```python
from build123d import *

# Parameters (mm, degrees)
ESQUISSE1_W             = 330
ESQUISSE1_H             = 220
BOSS_EXTRU_1_DEPTH      = 6
ESQUISSE3_W             = 20
ESQUISSE3_H             = 6
ESQUISSE3_W_2           = 30
ESQUISSE3_W_3           = 6
ESQUISSE3_H_2           = 10
ENL_V_MAT_EXTRU_2_DEPTH = 6
ESQUISSE4_R             = 1.4
ENL_V_MAT_EXTRU_3_DEPTH = 6


with BuildPart() as part:
    # Esquisse1 → Boss.-Extru.1 (new body)
    with BuildSketch(Plane.XY):
        Rectangle(ESQUISSE1_W, ESQUISSE1_H)
    extrude(amount=BOSS_EXTRU_1_DEPTH)

    # Esquisse3 → Enlèv. mat.-Extru.2 (cut)
    with BuildSketch(Plane.XY.offset(6)):
        with Locations((-125, 107)):
            Rectangle(ESQUISSE3_W, ESQUISSE3_H)
        with Locations((-50, 107)):
            Rectangle(ESQUISSE3_W_2, ESQUISSE3_H)
        with Locations((-162, 45)):
            Rectangle(ESQUISSE3_W_3, ESQUISSE3_H_2)
        with Locations((50, 107)):
            Rectangle(ESQUISSE3_W_2, ESQUISSE3_H)
        with Locations((-162, 85)):
            Rectangle(ESQUISSE3_W_3, ESQUISSE3_H_2)
        with Locations((162, 85)):
            Rectangle(ESQUISSE3_W_3, ESQUISSE3_H_2)
        with Locations((162, 45)):
            Rectangle(ESQUISSE3_W_3, ESQUISSE3_H_2)
        with Locations((125, 107)):
            Rectangle(ESQUISSE3_W, ESQUISSE3_H)
        with Locations((125, -107)):
            Rectangle(ESQUISSE3_W, ESQUISSE3_H)
        with Locations((50, -107)):
            Rectangle(ESQUISSE3_W_2, ESQUISSE3_H)
        with Locations((162, -45)):
            Rectangle(ESQUISSE3_W_3, ESQUISSE3_H_2)
        with Locations((162, -85)):
            Rectangle(ESQUISSE3_W_3, ESQUISSE3_H_2)
        with Locations((-162, -85)):
            Rectangle(ESQUISSE3_W_3, ESQUISSE3_H_2)
        with Locations((-162, -45)):
            Rectangle(ESQUISSE3_W_3, ESQUISSE3_H_2)
        with Locations((-50, -107)):
            Rectangle(ESQUISSE3_W_2, ESQUISSE3_H)
        with Locations((-125, -107)):
            Rectangle(ESQUISSE3_W, ESQUISSE3_H)
    extrude(amount=-ENL_V_MAT_EXTRU_2_DEPTH, mode=Mode.SUBTRACT)

    # Esquisse4 → Enlèv. mat.-Extru.3 (cut)
    with BuildSketch(Plane.XY.offset(6)):
        with Locations((-102.5, 107)):
            Circle(ESQUISSE4_R)
        with Locations((-77.5, 107)):
            Circle(ESQUISSE4_R)
        with Locations((-17.5, 107)):
            Circle(ESQUISSE4_R)
        with Locations((-162, 72.5)):
            Circle(ESQUISSE4_R)
        with Locations((-162, 57.5)):
            Circle(ESQUISSE4_R)
        with Locations((162, 57.5)):
            Circle(ESQUISSE4_R)
        with Locations((162, 72.5)):
            Circle(ESQUISSE4_R)
        with Locations((17.5, 107)):
            Circle(ESQUISSE4_R)
        with Locations((77.5, 107)):
            Circle(ESQUISSE4_R)
        with Locations((102.5, 107)):
            Circle(ESQUISSE4_R)
        with Locations((102.5, -107)):
            Circle(ESQUISSE4_R)
        with Locations((77.5, -107)):
            Circle(ESQUISSE4_R)
        with Locations((17.5, -107)):
            Circle(ESQUISSE4_R)
        with Locations((162, -72.5)):
            Circle(ESQUISSE4_R)
        with Locations((162, -57.5)):
            Circle(ESQUISSE4_R)
        with Locations((-162, -57.5)):
            Circle(ESQUISSE4_R)
        with Locations((-162, -72.5)):
            Circle(ESQUISSE4_R)
        with Locations((-17.5, -107)):
            Circle(ESQUISSE4_R)
        with Locations((-77.5, -107)):
            Circle(ESQUISSE4_R)
        with Locations((-102.5, -107)):
            Circle(ESQUISSE4_R)
    extrude(amount=-ENL_V_MAT_EXTRU_3_DEPTH, mode=Mode.SUBTRACT)


solid = part.part
```
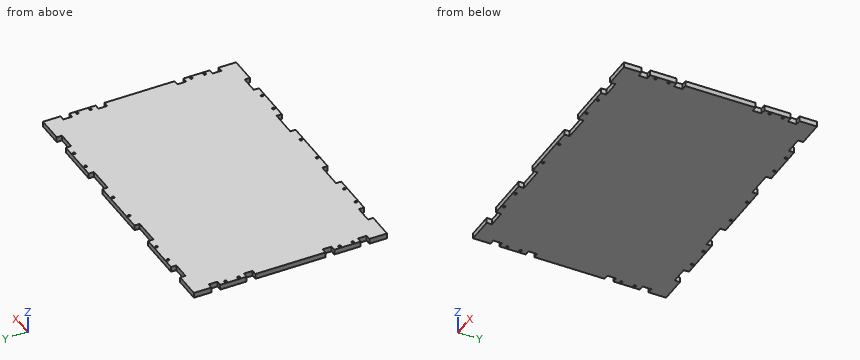
Source: CAD feature listing. Evaluate the final solid. Frame: model axes, mm. Coordinates: 2 decimals unless noted, no trailing zeros. Order: outer loops, then holes, each group sorted by start corner. A loop starts at its lowest first (then second) coordinate and runs counter-clockwise, first axis right, second up. Notation, with made-up numbers: M 6,6 L 22,6 A28 ccw 22,33 Z; hole C -30,87 d2. An arc over 180 degrees is marked long. Write each question's results on one line, items separated by ' | '. Start each with the question number.
1) Line query: line 1 (Y direction, x = 17.5, z = 4.25); line 2 (Y direction, x = 132.5, z = 5.65); line 3 (X direction, y = -72, z = 3.2). Output: solid intervals per line, ascending. Write a range as from..to.
2) Section query A-A (x = -119.5). Return the cut outline in (y, z), plus the area to 3 significant figures.
3) Section query B-B (z = 0.9). Give the number of separate pieces and of enclosed holes in the cut face, plus the area to 3 significant figures.
4) Contact query for flat-ended pins moving along their axis: pin 1 Ø3 at (x, z) = (49.5, 3.5) entering from -Y; pin 2 Ø3 at (x, z) = (-54.5, 3.5) entering from +Y; pin 3 Ø1.8 at (y, z) = (87.5, 4.5) entering from +X. Output: stop coordinate, or through.
Answers:
1) line 1: y = -110..-108.4, -105.6..105.6, 108.4..110 | line 2: y = -104..104 | line 3: x = -165..-163.31, -160.69..160.69, 163.31..165
2) outline: M -104,0 L 104,0 L 104,6 L -104,6 Z | area: 1,250 mm^2
3) separate pieces: 1 | enclosed holes: 20 | area: 70,800 mm^2
4) pin 1: stops at y = -104 | pin 2: stops at y = 104 | pin 3: stops at x = 159
